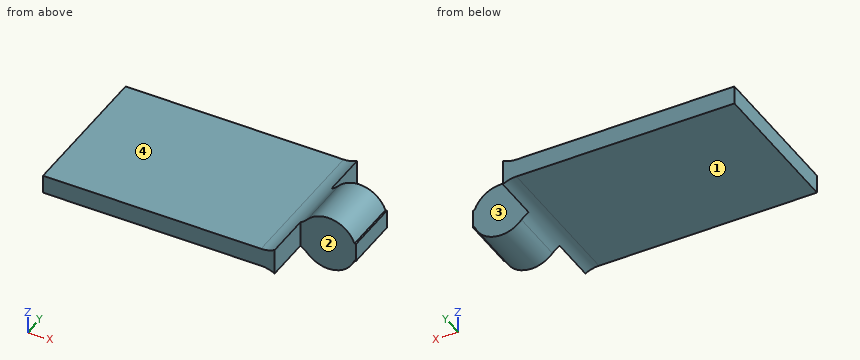
```python
from build123d import *

# Parameters (mm, degrees)
F0_W     = 3
F0_H     = 6
F3_DEPTH = 1
F4_D     = 1
F6_R     = 3


with BuildPart() as f2:
    # F0 (on Top) → F2 (revolve)
    with BuildSketch(Plane.XY):
        with Locations((1.5, 8)):
            Rectangle(F0_W, F0_H)
    revolve(axis=Axis((0, 8, 0), (0, -1, 0)))

    # F4 (through all)
    with Locations(Plane.XZ):
        with Locations((0, 0)):
            Hole(F4_D / 2)


with BuildPart() as f3:
    # F0 (on Top) → F3 (new body, symmetric)
    with BuildSketch(Plane.XY):
        Polygon((-28, 16), (-28, 0), (-3, 0), (-3, 5), (0, 5), (0, 11), (-3, 11), (-3, 16), align=None)
        with Locations((1.5, 8)):
            Rectangle(F0_W, F0_H)
    extrude(amount=F3_DEPTH, both=True)


with BuildPart() as f2_1:
    add(f2.part)

    # F5: union F3
    add(f3.part)

    # F6 (call 1 of 2: OpenCascade refuses the feature's edges together)
    f6_edges = [f2_1.edges().sort_by_distance(p)[0] for p in [
        (-2.828427, 8, 1),
    ]]
    fillet(f6_edges, radius=F6_R)

    # F6#2 (call 2 of 2)
    f6_2_edges = [f2_1.edges().sort_by_distance(p)[0] for p in [
        (-2.828427, 8, -1),
    ]]
    fillet(f6_2_edges, radius=F6_R)


solid = f2_1.part
```
Could you check a few things on this model? Use its own coordinates, in mm. Face numbers are marked on the shaded views. A direction names the side the tool comes from. Give positions to 0.01 mm unless a question says otherwise; leave off trailing zeros. Order: outer loops, then holes, each group sorted by start corner. A loop starts at its lowest first (then second) coordinate and runs counter-clockwise, first axis right, second up.
Q1. If I drill on line 1 along Y through (x, z) = (0.5, 1.35); line 2 along Z through (x, y) = (-13, 5); line 3 along X through (y, z) = (13, -0.3), over which ranges is the centre line in solid material (lowest first)?
Q2. Suppose I cut it at C-C, the plane x = -19.5. Write out the boundary of the cut face in (y, z).
Q3. Suppose I cut it at A-A, the plane z = -0.2. Write out the boundary of the cut face in (x, y), and give its area (3 significant figures).
Q4. Suppose I cut it at D-D, the plane y = 11.5. Write out the boundary of the cut face in (x, z).
Q5. For the marked faces 1, 2, 3 and 4, which set-ups out of +Z, -Z, +X, -X, +Y, -Y let a thin tool reach every point of the face, with its end or its side?
Q6. I'm going to push flat-ended pins straight in: P1, Ø1, axis at x = -3.5, y = 10.5, coming from the -Z side; P2, Ø2, axis at y = 3, z = 0.5, coming from the +X side. Where does each tip first touch, or does it pass through?
Q7. Suppose I cut it at B-B, the plane y = 7.5. Write out the boundary of the cut face in (x, z).
Solution:
1. line 1: y = 5 to 11
1. line 2: z = -1 to 1
1. line 3: x = -28 to -3
2. outline: (0, -1) - (16, -1) - (16, 1) - (0, 1) - close
3. outline: (-28, 0) - (-3, 0) - (-3, 5) - (3, 5) - (3, 11) - (-3, 11) - (-3, 16) - (-28, 16) - close
3. area: 436 mm2
4. outline: (-28, -1) - (-4.47, -1) arc R3 cw to (-3, -1.39) - (-3, 1.39) arc R3 cw to (-4.47, 1) - (-28, 1) - close
5. face 1: -Z, -X, +Y, -Y
5. face 2: +Z, -Z, +X, -Y
5. face 3: +Z, -Z, +X, +Y
5. face 4: +Z, -X, +Y, -Y
6. P1: stops at z = -1.39
6. P2: stops at x = -3
7. outline: (-28, -1) - (-4.47, -1) arc R3 cw to (-2.24, -2) arc R3 ccw to (2.83, -1) - (3, -1) - (3, 1) - (2.83, 1) arc R3 ccw to (-2.24, 2) arc R3 cw to (-4.47, 1) - (-28, 1) - close
